from build123d import *

# Parameters (mm, degrees)
IZIM1_W                     = 27.91
IZIM1_H                     = 26.13
IZIM1_W_2                   = 25.91
IZIM1_H_2                   = 24.13
Y_KSEKLIK_EKSTR_ZYON1_DEPTH = 2.2
RADYUS1_R                   = 3
Y_KSEKLIK_EKSTR_ZYON2_DEPTH = 0.252
IZIM3_R                     = 13.875
Y_KSEKLIK_EKSTR_ZYON3_DEPTH = 6.35


with BuildPart() as part:
    # Çizim1 → Yükseklik-Ekstrüzyon1 (new body)
    with BuildSketch(Plane(origin=(0, 0, 0), x_dir=(1, 0, 0), z_dir=(0, 1, 0))):
        Rectangle(IZIM1_W, IZIM1_H)
        Rectangle(IZIM1_W_2, IZIM1_H_2, mode=Mode.SUBTRACT)
    extrude(amount=Y_KSEKLIK_EKSTR_ZYON1_DEPTH)

    # Radyus1
    radyus1_edges = [part.edges().sort_by_distance(p)[0] for p in [
        (12.955, 1.1, 12.065),
        (12.955, 1.1, -12.065),
        (-12.955, 1.1, -12.065),
        (-12.955, 1.1, 12.065),
        (-13.955, 1.1, -13.065),
        (13.955, 1.1, -13.065),
        (13.955, 1.1, 13.065),
        (-13.955, 1.1, 13.065),
    ]]
    fillet(radyus1_edges, radius=RADYUS1_R)

    # Çizim2 → Yükseklik-Ekstrüzyon2 (add)
    with BuildSketch(Plane.XZ):
        with BuildLine():
            Line((10.955, 13.065), (-10.955, 13.065))
            ThreePointArc((-10.955, 13.065), (-13.076320344, 12.186320344), (-13.955, 10.065))
            Line((-13.955, 10.065), (-13.955, -10.065))
            ThreePointArc((-13.955, -10.065), (-13.076320344, -12.186320344), (-10.955, -13.065))
            Line((-10.955, -13.065), (10.955, -13.065))
            ThreePointArc((10.955, -13.065), (13.076320344, -12.186320344), (13.955, -10.065))
            Line((13.955, -10.065), (13.955, 10.065))
            ThreePointArc((13.955, 10.065), (13.076320344, 12.186320344), (10.955, 13.065))
        make_face()
    extrude(amount=Y_KSEKLIK_EKSTR_ZYON2_DEPTH)

    # Çizim3 → Yükseklik-Ekstrüzyon3 (add)
    with BuildSketch(Plane.XZ.offset(0.252)):
        with Locations(Location((0, 0, 0), (0, 0, 70.325694482))):
            Circle(IZIM3_R)
    extrude(amount=Y_KSEKLIK_EKSTR_ZYON3_DEPTH)


solid = part.part
Input: part model. Units: mm. Frame: model coordinates. A direction names the side the tool comes from. Coordinates: 2 decimals unless noted, no trailing zeros. Order: outer loops, then holes, each group sorted by start corner. A loop starts at its lowest first (then second) coordinate and runs counter-clockwise, first axis right, second up. Notation, with made-up numbers: M 9.25,52.25 L 51.25,52.25 A19 cw 51.25,73.25 Z; hole C -21.75,-17 d3. An arc over 180 degrees is marked long. One line per question, with ' | ' between items.
Item 1: Section C-C (z = 0). Output: boundary loops of the cut face in (x, y) (3 decimals), then the cut area to 3 significant figures.
Geometry results:
outline: M -13.955,-0.252 L -13.875,-0.252 L -13.875,-6.602 L 13.875,-6.602 L 13.875,-0.252 L 13.955,-0.252 L 13.955,2.2 L 12.955,2.2 L 12.955,0 L -12.955,0 L -12.955,2.2 L -13.955,2.2 Z | area: 188 mm^2
Item 2: Ray query, line 1 along X through (y, z) = (1.5, 0) (3 decimals); line 2 along Y through (x, z) = (-12.25, 1.75); line 3 along X through (y, z) = (1.75, 9.5) (3 decimals). Return the intervals inside material, ascending.
Geometry results:
line 1: x = -13.955 to -12.955, 12.955 to 13.955 | line 2: y = -6.6 to 0 | line 3: x = -13.955 to -12.923, 12.923 to 13.955
Item 3: Section A-A (x = 0). Output: boundary loops of the cut face in (y, z) (3 decimals).
Geometry results:
outline: M -6.602,-13.875 L -0.252,-13.875 L -0.252,-13.065 L 2.2,-13.065 L 2.2,-12.065 L 0,-12.065 L 0,12.065 L 2.2,12.065 L 2.2,13.065 L -0.252,13.065 L -0.252,13.875 L -6.602,13.875 Z
Item 4: Section D-D (y = -4.75). Output: boundary loops of the cut face in (x, z) (3 decimals).
Geometry results:
outline: C 0,0 d27.75
Item 5: Section B-B (y = 1). Output: boundary loops of the cut face in (x, z) (3 decimals).
Geometry results:
outline: M -13.955,-10.065 A3 ccw -10.955,-13.065 L 10.955,-13.065 A3 ccw 13.955,-10.065 L 13.955,10.065 A3 ccw 10.955,13.065 L -10.955,13.065 A3 ccw -13.955,10.065 Z; hole M -12.955,-9.065 A3 ccw -9.955,-12.065 L 9.955,-12.065 A3 ccw 12.955,-9.065 L 12.955,9.065 A3 ccw 9.955,12.065 L -9.955,12.065 A3 ccw -12.955,9.065 Z
Item 6: Draft query along X for faces 1 (the cylindrical face through (13.05, 0.99, -12.21)), 2 (the flat face through (12.955, 1, 0)), 3 (the flat face through (0, -6.602, 0)), 4 (the cylindrical face through (-12.05, 1.12, -11.21)). Return one class per face: released by +X, released by -X, zero draft, split by the parting line, or undercut.
Geometry results:
face 1: released by +X | face 2: undercut | face 3: zero draft | face 4: undercut
Item 7: Pin query (flat end, axial travel): pin 1 (2 mm diameter, centred on x = 3.5, y = 1, fed in from +Z) (3 decimals); pin 2 (0.6 mm diameter, centred on x = 0.5, z = 13.5, fed in from +Y); pin 3 (5 mm diameter, centred on x = -2, z = 2.5, fed in from +Y). Return the tip coordinate at first contact, or that it passes through.
Geometry results:
pin 1: stops at z = 13.065 | pin 2: stops at y = -0.25 | pin 3: stops at y = 0
Item 8: Reachability of faces 5 (the flat face through (0, 1, -13.065)), 6 (the cylindrical face through (12.05, 1.12, 11.21)), 7 (the cylindrical face through (-13.562, -3.383, 2.931)), 8 (the flat face through (0.1, -0.252, 13.4)) from +Z, -Z, +X, -X, +Y, -Y: full face, straight path, thin tool, end or side. Return the list, or none.
Geometry results:
face 5: -Z, +X, -X, +Y | face 6: +Y | face 7: -Y | face 8: +Z, +X, -X, +Y
